```python
from build123d import *

# Parameters (mm, degrees)
SKETCH1_R           = 6.35
SKETCH1_R_2         = 9.525
BOSS_EXTRUDE1_DEPTH = 14.615
CUT_EXTRUDE1_DEPTH  = 91.641086881
SKETCH4_W           = 13.23
SKETCH4_H           = 38
CUT_EXTRUDE2_DEPTH  = 104.718600248
CUT_EXTRUDE3_DEPTH  = 6


with BuildPart() as part:
    # Sketch1 → Boss-Extrude1 (new, symmetric)
    with BuildSketch(Plane(origin=(0, 0, 0), x_dir=(0, 0, -1), z_dir=(1, 0, 0))):
        with BuildLine():
            Line((0, -22), (60, -22))
            Line((60, -22), (60, 14))
            ThreePointArc((60, 14), (24.306087072, 24.928324713), (0, 53.260247211))
            ThreePointArc((0, 53.260247211), (-16.383810232, 60.832127863), (-26.61523279, 45.963348263))
            Line((-26.61523279, 45.963348263), (-21.894870769, -2.148169925))
            ThreePointArc((-21.894870769, -2.148169925), (-14.777351956, -16.298155392), (0, -22))
        make_face()
        with Locations((-12.68213321, 47.330365488)):
            Circle(SKETCH1_R, mode=Mode.SUBTRACT)
        Circle(SKETCH1_R_2, mode=Mode.SUBTRACT)
    extrude(amount=BOSS_EXTRUDE1_DEPTH, both=True)

    # Sketch2 → Cut-Extrude1 (cut, through all)
    with BuildSketch(Plane(origin=(14.615, 0, 0), x_dir=(0, 0, -1), z_dir=(1, 0, 0))):
        with BuildLine():
            Line((38, 0), (60, 0))
            ThreePointArc((60, 0), (64, -4), (60, -8))
            Line((60, -8), (38, -8))
            ThreePointArc((38, -8), (34, -4), (38, 0))
        make_face()
    extrude(amount=-CUT_EXTRUDE1_DEPTH, mode=Mode.SUBTRACT)

    # Sketch4 → Cut-Extrude2 (cut, through all)
    with BuildSketch(Plane.XZ.offset(22)):
        with Locations((0, -41)):
            Rectangle(SKETCH4_W, SKETCH4_H)
    extrude(amount=-CUT_EXTRUDE2_DEPTH, mode=Mode.SUBTRACT)

    # Sketch5 → Cut-Extrude3 (cut)
    with BuildSketch(Plane(origin=(14.615, 0, 0), x_dir=(0, 0, -1), z_dir=(1, 0, 0))):
        with BuildLine():
            Line((3.099615742, 36.750365488), (10.675895531, 36.750365488))
            ThreePointArc((10.675895531, 36.750365488), (4.729057579, 44.611575605), (0, 53.260247211))
            ThreePointArc((0, 53.260247211), (-16.383810232, 60.832127863), (-26.61523279, 45.963348263))
            Line((-26.61523279, 45.963348263), (-25.360971776, 33.179497931))
            ThreePointArc((-25.360971776, 33.179497931), (-10.316803002, 28.478171637), (3.099615742, 36.750365488))
        make_face()
    cut_extrude3 = extrude(amount=-CUT_EXTRUDE3_DEPTH, mode=Mode.SUBTRACT)

    # Mirror1: Cut-Extrude3 across plane
    add(cut_extrude3.mirror(Plane(origin=(0, 0, 0), x_dir=(0, 0, 1), z_dir=(1, 0, 0))), mode=Mode.SUBTRACT)


solid = part.part
```
The model under review builds one solid part; all positions refer to its coordinate system, in mm. A direction names the side the tool comes from. Round coordinates to 2 decimals unless told otherwise and drop trailing zeros. Loops run counter-clockwise (first coordinate to the right, second up) from the corner with the lowest first, then second, coordinate; pieces in that order, holes last.
1) Tool access review of faces 5 (the face through (11.66, 28.45, 10.54)), 6 (the face through (11, 0, -49)), 7 (the face through (-11.66, 28.45, 10.54)): name each direction out of +Z, -Z, +X, -X, +Y, -Y from which nothing blocks a thin tool from reaching the whole face with its end or side.
Values follow:
face 5: +X, +Y
face 6: -Z, +X, -X
face 7: -X, +Y
2) Consider section D-D on z = -40.5. State the section outline as (x, y) points (3 decimals).
Values follow:
outline: (-14.615, -22) - (-6.615, -22) - (-6.615, -8) - (-14.615, -8) - close; (-14.615, 0) - (-6.615, 0) - (-6.615, 17.203) - (-14.615, 17.203) - close; (6.615, -22) - (14.615, -22) - (14.615, -8) - (6.615, -8) - close; (6.615, 0) - (14.615, 0) - (14.615, 17.203) - (6.615, 17.203) - close
3) Wall thickness on line 1 along Y through (x, z) = (2.25, 11.5) (3 decimals); line 2 along Y through (x, z) = (12, -51.5); line 3 along X through (y, z) = (39, -6) (3 decimals): over which ranges is each line inside the solid? List them lowest first.
Values follow:
line 1: y = -18.755 to 41.091, 53.569 to 61.28
line 2: y = -22 to -8, 0 to 14.67
line 3: x = -8.615 to 8.615
4) Consider section C-C on x = -0.75. State the section outline as (y, z) points (3 decimals).
Values follow:
outline: (-22, -22) - (26.507, -22) arc R67 cw to (53.26, 0) arc R14 ccw to (45.963, 26.615) - (-2.148, 21.895) arc R22 ccw to (-22, 0) - close; hole circle Ø19.05 at (0, 0); hole circle Ø12.7 at (47.33, 12.682)
5) Consider section B-B on z = -29. State the section outline as (x, y) points (3 decimals).
Values follow:
outline: (-14.615, -22) - (-6.615, -22) - (-6.615, 22.124) - (-14.615, 22.124) - close; (6.615, -22) - (14.615, -22) - (14.615, 22.124) - (6.615, 22.124) - close
6) The part is to be moulded in two halves that separate along Y. For faces 1 (the face through (-0.121, 51.622, 17.362)), 2 (the face through (-11, 0, -49)), 3 (the face through (6.615, 2, -41)), 4 (the face through (12, 36.75, -7)), say which applies: pulls with the +Y half, pulls with the -Y half, needs draft (parallel to the pull), parting line crosses it, or undercut.
Values follow:
face 1: undercut
face 2: undercut
face 3: needs draft
face 4: pulls with the +Y half
7) Consider section A-A on y = -7. State the section outline as (x, z) points (3 decimals), then the cut area to 3 significant figures.
Values follow:
outline: (-14.615, -35.354) - (-6.615, -35.354) - (-6.615, -22) - (6.615, -22) - (6.615, -35.354) - (14.615, -35.354) - (14.615, -6.46) - (-14.615, -6.46) - close; (-14.615, 6.46) - (14.615, 6.46) - (14.615, 20.857) - (-14.615, 20.857) - close
area: 1,090 mm2
8) Clearance check with flat-ended pins moving along their axes: P1, Ø12, axis at x = 11, z = -40.5, coming from the +Y side; P2, Ø1.5, axis at x = 5.5, z = 11.5, coming from the -Y side; P3, Ø20.5, axis at y = 47.33, z = 12.68, coming from the -X side (3 decimals). State where each tip first meets the part, or that it passes through.
Values follow:
P1: stops at y = 19.45
P2: stops at y = -19.19
P3: stops at x = -8.615
